Input: part model. Units: mm. Frame: model coordinates. Face numbers are marked on the shaded views. A direction names the side the tool comes from. Coordinates: 2 decimals unless noted, no trailing zeros. Loops run counter-clockwise (first coordinate to the right, second up) from the corner with the lowest first, then second, coordinate; pieces in that order, holes last.
```python
from build123d import *

# Parameters (mm, degrees)
CROQUIS1_W              = 20
CROQUIS1_H              = 22
SALIENTE_EXTRUIR1_DEPTH = 1
CROQUIS2_W              = 8
CROQUIS2_H              = 1
SALIENTE_EXTRUIR2_DEPTH = 20
CROQUIS3_R              = 1.5
CORTAR_EXTRUIR1_DEPTH   = 33.015621187
CROQUIS4_R              = 1.5
SALIENTE_EXTRUIR3_DEPTH = 8
REDONDEO1_R             = 6


with BuildPart() as part:
    # Croquis1 → Saliente-Extruir1 (new body)
    with BuildSketch(Plane(origin=(0, 0, 0), x_dir=(1, 0, 0), z_dir=(0, 1, 0))):
        Rectangle(CROQUIS1_W, CROQUIS1_H)
    extrude(amount=SALIENTE_EXTRUIR1_DEPTH)

    # Croquis2 → Saliente-Extruir2 (add)
    with BuildSketch(Plane(origin=(0, 1, 0), x_dir=(1, 0, 0), z_dir=(0, 1, 0))):
        with Locations((0, -10.5)):
            Rectangle(CROQUIS2_W, CROQUIS2_H)
        with Locations((0, 10.5)):
            Rectangle(CROQUIS2_W, CROQUIS2_H)
    extrude(amount=SALIENTE_EXTRUIR2_DEPTH)

    # Croquis3 → Cortar-Extruir1 (cut, through all)
    with BuildSketch(Plane.XY.offset(11)):
        with Locations((0, 8)):
            Circle(CROQUIS3_R)
        with BuildLine():
            Line((-4, 8), (-13.08141652, 8))
            Line((-13.08141652, 8), (-13.08141652, 28.561512487))
            Line((-13.08141652, 28.561512487), (15.549721507, 28.561512487))
            Line((15.549721507, 28.561512487), (15.549721507, 8))
            Line((15.549721507, 8), (4, 8))
            ThreePointArc((4, 8), (0, 12), (-4, 8))
        make_face()
    extrude(amount=-CORTAR_EXTRUIR1_DEPTH, mode=Mode.SUBTRACT)

    # Croquis4 → Saliente-Extruir3 (add)
    with BuildSketch(Plane.XZ):
        with Locations(Location((0, 0, 0), (0, 0, 270))):
            Circle(CROQUIS4_R)
    extrude(amount=SALIENTE_EXTRUIR3_DEPTH)

    # Redondeo1
    redondeo1_edges = [part.edges().sort_by_distance(p)[0] for p in [
        (-10, 0.5, -11),
        (-10, 0.5, 11),
        (10, 0.5, -11),
        (10, 0.5, 11),
    ]]
    fillet(redondeo1_edges, radius=REDONDEO1_R)


solid = part.part
```
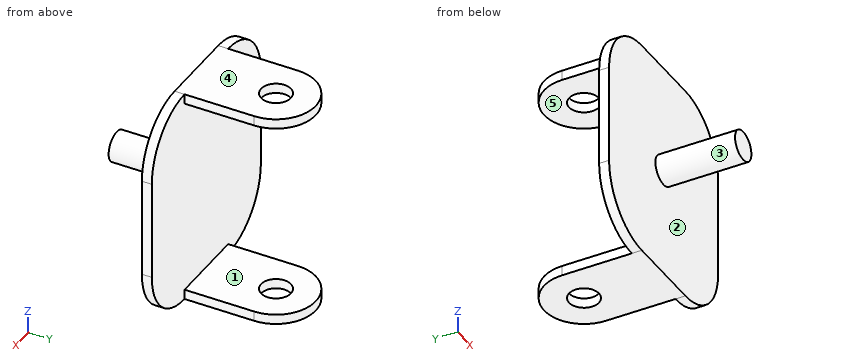
Item 1: Section query C-C (y = 10.75). Output: boundary loops of the cut face in (x, z).
Result:
outline: (-2.9, -11) - (2.9, -11) - (2.9, -10) - (-2.9, -10) - close; (-2.9, 10) - (2.9, 10) - (2.9, 11) - (-2.9, 11) - close
Item 2: Reachability of the marked faces 4 and 5 from +Z, -Z, +X, -X, +Y, -Y: full face, straight path, thin tool, end or side. Return the list, or none.
Result:
face 4: +Z, +X, -X, +Y, -Y
face 5: +X, -X, +Y
Item 3: Line query: L1, parallel to Z at x = 1.25, y = 9.5; L2, parallel to Y at x = 0, z = 10.6; L3, parallel to Y at x = 8, z = 4.75. Output: solid intervals per line, ascending.
Result:
L1: z = -11 to -10, 10 to 11
L2: y = 0 to 6.5, 9.5 to 12
L3: y = 0 to 1
Item 4: Mould query, pull axis Z, two halves, no side actions, for the marked faces 1, 2 and 3. Classes: +Z half, -Z half, draft (parallel to the pull), parting line (faces both ways), or undercut.
Result:
face 1: undercut
face 2: draft
face 3: parting line
Item 5: Section query D-D (y = 0.5). Output: boundary loops of the cut face in (x, z).
Result:
outline: (-10, -5) arc R6 ccw to (-4, -11) - (4, -11) arc R6 ccw to (10, -5) - (10, 5) arc R6 ccw to (4, 11) - (-4, 11) arc R6 ccw to (-10, 5) - close
Item 6: Contact query for flat-ended pins moving along their axis: P1, Ø10, axis at x = -3.5, z = -2, coming from the +Y side; P2, Ø1.5, axis at x = -4.5, y = -2, coming from the -Z side; P3, Ø12, axis at x = 5, z = -8, coming from the -Y side; P4, Ø0.8, axis at y = 4.5, z = -10.5, coming from the +X side. Output: stop coordinate, or through.
Result:
P1: stops at y = 1
P2: passes through
P3: stops at y = 0
P4: stops at x = 4
Item 7: Section query A-A (x = 0). Output: boundary loops of the cut face in (y, z), then the cut area to 3 significant figures.
Result:
outline: (-8, -1.5) - (0, -1.5) - (0, -11) - (6.5, -11) - (6.5, -10) - (1, -10) - (1, 10) - (6.5, 10) - (6.5, 11) - (0, 11) - (0, 1.5) - (-8, 1.5) - close; (9.5, -11) - (12, -11) - (12, -10) - (9.5, -10) - close; (9.5, 10) - (12, 10) - (12, 11) - (9.5, 11) - close
area: 62.0 mm2
Item 8: Section query B-B (z = 0). Output: boundary loops of the cut face in (x, y).
Result:
outline: (-10, 0) - (-1.5, 0) - (-1.5, -8) - (1.5, -8) - (1.5, 0) - (10, 0) - (10, 1) - (-10, 1) - close
